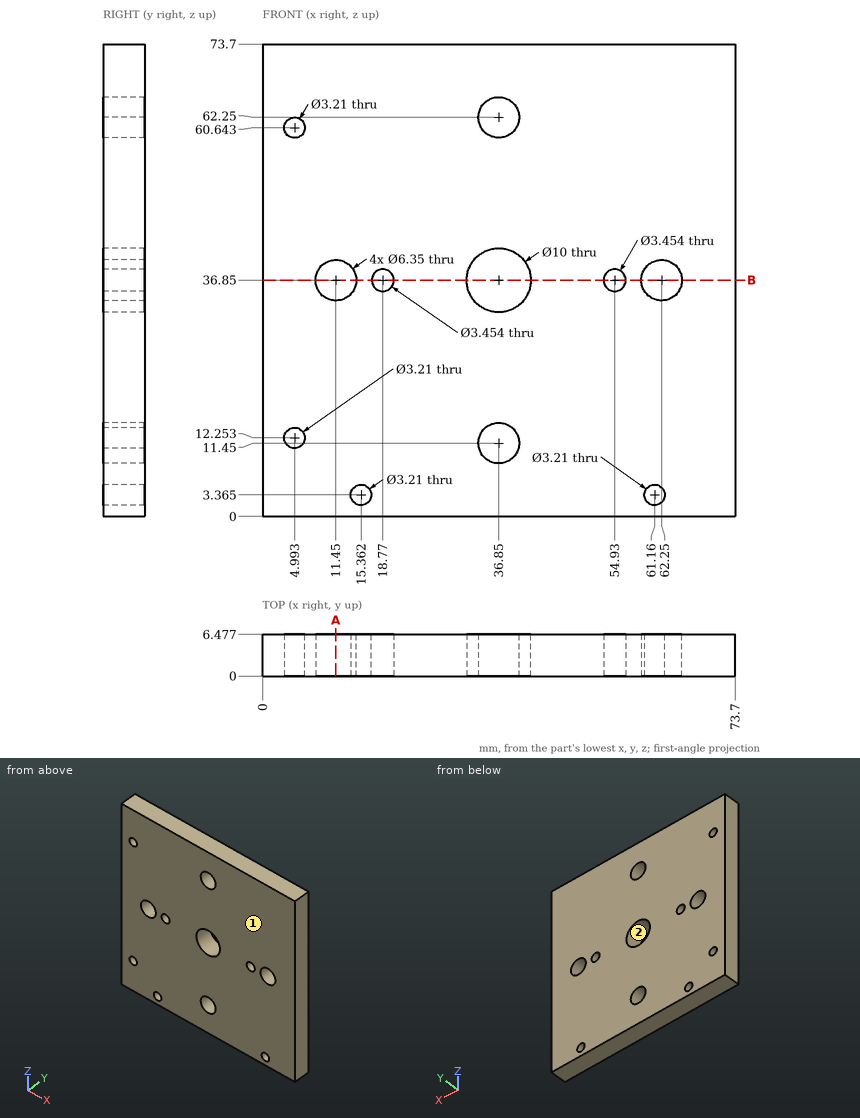
Part print with two shaded views. Sizes in mm from the minimum x, y, z corner. Give positions to 0.01 mm unless a question says otherwise; leave off trailing zeros. Loops run counter-clockwise (first coordinate to the right, second up) from the corner with the lowest first, then second, coordinate; pieces in that order, holes last. Notation, with made-up numbers: (-17.75, 2) - (25.25, 2) arc R28 cw to (25.25, 21) - close; hole circle Ø6 at (14.5, 55). An arc over 180 degrees is marked (long way). Put each result on its own line as item: value.
Q1. Slice it at B-B (z = 36.85). Give the number of separate pieces and of enclosed holes in the cut face.
Filled in:
separate pieces: 6
enclosed holes: 0
Q2. Mould opens along Z. For the marked faces 1 and 2 say: pulls with the +Z half, pulls with the -Z half, needs draft (parallel to the pull), parting line crosses it, or undercut.
Filled in:
face 1: needs draft
face 2: undercut
Q3. Slice it at A-A (x = 11.45). Give the cut face in (y, z) (1 decimal).
Filled in:
outline: (0, 0) - (6.5, 0) - (6.5, 33.7) - (0, 33.7) - close; (0, 40) - (6.5, 40) - (6.5, 73.7) - (0, 73.7) - close
Q4. Probe line 1 along Z through (x, y) = (11.45, 3.75) (1 decimal); line 2 along Z through (x, y) = (55, 4) (1 decimal). List the from-to ranges inside material, lowest first.
Filled in:
line 1: z = 0 to 33.7, 40 to 73.7
line 2: z = 0 to 35.1, 38.6 to 73.7
